The model under review builds one solid part; all positions refer to its coordinate system, in mm. Face numbers are marked on the shaded views. A direction names the side the tool comes from. Give positions to 0.01 mm unless a question says otherwise; leave off trailing zeros. Order: outer loops, then holes, each group sorted by start corner. A loop starts at its lowest first (then second) coordinate and runs counter-clockwise, first axis right, second up.
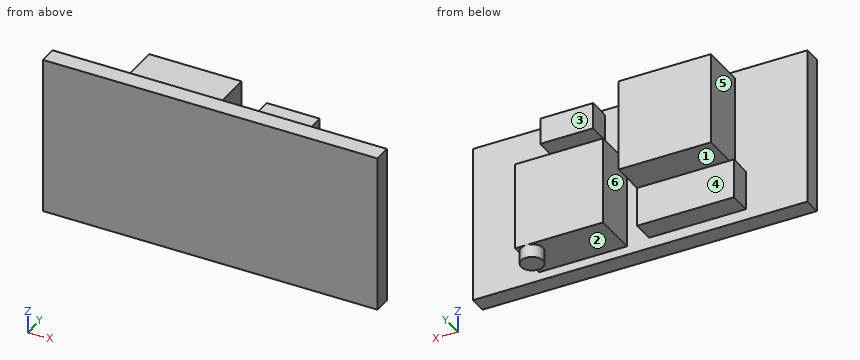
```python
from build123d import *

# Parameters (mm, degrees)
SKETCH1_W           = 38
SKETCH1_H           = 18
BOSS_EXTRUDE1_DEPTH = 2
SKETCH2_W           = 6
SKETCH2_H           = 3
SKETCH2_W_2         = 11
SKETCH2_H_2         = 4.5
BOSS_EXTRUDE2_DEPTH = 2.5
SKETCH3_W           = 10.5
SKETCH3_H           = 10.5
SKETCH3_W_2         = 10
SKETCH3_H_2         = 10
BOSS_EXTRUDE3_DEPTH = 5
SKETCH4_R           = 1.25
BOSS_EXTRUDE4_DEPTH = 1.5


with BuildPart() as part:
    # Sketch1 → Boss-Extrude1 (new body)
    with BuildSketch(Plane(origin=(0, 0, 0), x_dir=(1, 0, 0), z_dir=(0, 1, 0))):
        Rectangle(SKETCH1_W, SKETCH1_H)
    extrude(amount=BOSS_EXTRUDE1_DEPTH)

    # Sketch2 → Boss-Extrude2 (add)
    with BuildSketch(Plane(origin=(0, 2, 0), x_dir=(1, 0, 0), z_dir=(0, 1, 0))):
        with Locations((7, -6.9)):
            Rectangle(SKETCH2_W, SKETCH2_H)
        with Locations((-6.5, 5.5)):
            Rectangle(SKETCH2_W_2, SKETCH2_H_2)
    extrude(amount=BOSS_EXTRUDE2_DEPTH)

    # Sketch3 → Boss-Extrude3 (add)
    with BuildSketch(Plane(origin=(0, 2, 0), x_dir=(1, 0, 0), z_dir=(0, 1, 0))):
        with Locations((-5.5, -3)):
            Rectangle(SKETCH3_W, SKETCH3_H)
        with Locations((6.5, 3)):
            Rectangle(SKETCH3_W_2, SKETCH3_H_2)
    extrude(amount=BOSS_EXTRUDE3_DEPTH)

    # Sketch4 → Boss-Extrude4 (add)
    with BuildSketch(Plane(origin=(0, 0, -8), x_dir=(-1, 0, 0), z_dir=(0, 0, -1))):
        with Locations(Location((-10.25, 5.75, 0), (0, 0, 180))):
            Circle(SKETCH4_R)
    extrude(amount=BOSS_EXTRUDE4_DEPTH)


solid = part.part
```
Item 1: Take a section at B-B (x = 2.5). Give the boundary of the cut face in (y, z).
Values found:
outline: (0, -9) - (2, -9) - (2, -8) - (7, -8) - (7, 2) - (2, 2) - (2, 9) - (0, 9) - close
Item 2: Clearance check with flat-ended pins moving along their axes: pin 1 Ø2 at (x, y) = (6, 3.5) entering from +Z; pin 2 Ø1.2 at (x, y) = (7, 3.5) entering from -Z; pin 3 Ø1.5 at (x, y) = (-5, 3.5) entering from -Z; pin 4 Ø10 at (x, z) = (-13, 1) entering from +Y. State where each tip first meets the part, or that it passes through.
Values found:
pin 1: stops at z = 8.4
pin 2: stops at z = -8
pin 3: stops at z = -7.75
pin 4: stops at y = 7
Item 3: For line 1 (X direction, y = 3.5, z = -5.5); line 2 (Z direction, x = -6, y = 2.75); line 3 (X direction, y = 3.5, z = 1.5), list the stretches that pass through material, from the lowest coordinate up.
Values found:
line 1: x = -12 to -1, 1.5 to 11.5
line 2: z = -7.75 to -3.25, -2.25 to 8.25
line 3: x = -10.75 to -0.25, 1.5 to 11.5
Item 4: For the marked faces 4, 5 and 6, list the 3-axis set-ups (+Z, -Z, +X, -X, +Y, -Y) from which the entire face can be reached by the end or side of a thin tool; tool diameter is ignored.
Values found:
face 4: -Z, -X, +Y
face 5: +Z, -X, +Y
face 6: +Z, -Z, +Y
Item 5: Take a section at A-A (y = 2.5). Give the boundary of the cut face in (x, z).
Values found:
outline: (-12, -7.75) - (-1, -7.75) - (-1, -3.25) - (-12, -3.25) - close; (-10.75, -2.25) - (-0.25, -2.25) - (-0.25, 8.25) - (-10.75, 8.25) - close; (1.5, -8) - (11.5, -8) - (11.5, 2) - (1.5, 2) - close; (4, 5.4) - (10, 5.4) - (10, 8.4) - (4, 8.4) - close
Item 6: Take a section at D-D (y = 1). Give the boundary of the cut face in (x, z), and give its area (3 significant figures).
Values found:
outline: (-19, -9) - (19, -9) - (19, 9) - (-19, 9) - close
area: 684 mm2
Item 7: Draft analysis for pull direction Z (two halves, no side actions). For the marked faces 1, 2 and 3, state which applies: released by +Z, released by -Z, zero draft, split by the parting line, or undercut.
Values found:
face 1: undercut
face 2: released by -Z
face 3: zero draft
Item 8: Take a section at C-C (z = 5). Give the boundary of the cut face in (x, y), and give its area (4 significant figures).
Values found:
outline: (-19, 0) - (19, 0) - (19, 2) - (-0.25, 2) - (-0.25, 7) - (-10.75, 7) - (-10.75, 2) - (-19, 2) - close
area: 128.5 mm2
